Input: part model. Units: mm. Frame: model coordinates. A direction names the side the tool comes from. Coordinates: 2 decimals unless noted, no trailing zeros. Order: outer loops, then holes, each group sorted by start corner. A loop starts at its lowest first (then second) coordinate and runs counter-clockwise, first axis right, second up.
from build123d import *

# Parameters (mm, degrees)
BOSS_EXTRUDE1_DEPTH = 100
FILLET1_R           = 1
SKETCH2_R           = 2.5
CUT_EXTRUDE1_DEPTH  = 102.7840852
CUT_EXTRUDE2_DEPTH  = 102.7840852


with BuildPart() as part:
    # Sketch1 → Boss-Extrude1 (new body)
    with BuildSketch(Plane.XY):
        Polygon((0, 0), (18, 0), (18, 3), (3, 3), (3, 9), (0, 9), align=None)
    extrude(amount=BOSS_EXTRUDE1_DEPTH)

    # Fillet1
    fillet1_edges = [part.edges().sort_by_distance(p)[0] for p in [
        (3, 9, 50),
        (3, 3, 50),
        (18, 3, 50),
    ]]
    fillet(fillet1_edges, radius=FILLET1_R)

    # Sketch2 → Cut-Extrude1 (cut, through all)
    with BuildSketch(Plane(origin=(0, 3, 0), x_dir=(1, 0, 0), z_dir=(0, 1, 0))):
        with Locations(Location((10.5, -25, 0), (0, 0, 180))):
            Circle(SKETCH2_R)
        with Locations(Location((10.5, -75, 0), (0, 0, 180))):
            Circle(SKETCH2_R)
    extrude(amount=-CUT_EXTRUDE1_DEPTH, mode=Mode.SUBTRACT)

    # Sketch3 → Cut-Extrude2 (cut, through all)
    with BuildSketch(Plane(origin=(0, 3, 0), x_dir=(1, 0, 0), z_dir=(0, 1, 0))):
        with BuildLine():
            Line((8, -72.5), (13, -72.5))
            ThreePointArc((13, -72.5), (15.5, -75), (13, -77.5))
            Line((13, -77.5), (8, -77.5))
            ThreePointArc((8, -77.5), (5.5, -75), (8, -72.5))
        make_face()
        with BuildLine():
            Line((8, -27.5), (13, -27.5))
            ThreePointArc((13, -27.5), (15.5, -25), (13, -22.5))
            Line((13, -22.5), (8, -22.5))
            ThreePointArc((8, -22.5), (5.5, -25), (8, -27.5))
        make_face()
    extrude(amount=-CUT_EXTRUDE2_DEPTH, mode=Mode.SUBTRACT)


solid = part.part
Item 1: Ray query, probe 1 along Z at (x, y) = (11.5, 2.25); probe 2 along Y at (x, z) = (9.5, 87). Return the intervals inside material, ascending.
Response values:
probe 1: z = 0 to 22.5, 27.5 to 72.5, 77.5 to 100
probe 2: y = 0 to 3
Item 2: Pin query (flat end, axial travel): pin 1 Ø10.5 at (x, z) = (12, 40) entering from +Y; pin 2 Ø3 at (y, z) = (6.5, 55) entering from +X. Return the tip coordinate at first contact, or that it passes through.
Response values:
pin 1: stops at y = 3
pin 2: stops at x = 3
Item 3: Cut plane D-D on x = 6.5. Return loops of the section in (y, z).
Response values:
outline: (0, 0) - (3, 0) - (3, 23) - (0, 23) - close; (0, 27) - (3, 27) - (3, 73) - (0, 73) - close; (0, 77) - (3, 77) - (3, 100) - (0, 100) - close
Item 4: Access query for faces 5 (the face through (10, 2, 72.5)), 6 (the face through (11, 3, 49)), 7 (the face through (6.9, 2.6, 100)). Directions: +Z, -Z, +X, -X, +Y, -Y. A direction counts if a zero-diameter tool reaches every point of the face in a straight line with its end or side. Return the directions, or none.
Response values:
face 5: +Y, -Y
face 6: +Z, -Z, +X, +Y
face 7: +Z, +X, -X, +Y, -Y
Item 5: Cut plane A-A on z = 25. Return loops of the section in (x, y).
Response values:
outline: (0, 0) - (5.5, 0) - (5.5, 3) - (4, 3) arc R1 cw to (3, 4) - (3, 8) arc R1 ccw to (2, 9) - (0, 9) - close; (15.5, 0) - (18, 0) - (18, 2) arc R1 ccw to (17, 3) - (15.5, 3) - close
Item 6: Cut plane B-B on x = 11.5. Return loops of the section in (y, z), then the cut area to 3 significant figures.
Response values:
outline: (0, 0) - (3, 0) - (3, 22.5) - (0, 22.5) - close; (0, 27.5) - (3, 27.5) - (3, 72.5) - (0, 72.5) - close; (0, 77.5) - (3, 77.5) - (3, 100) - (0, 100) - close
area: 270 mm2
Item 7: Draft query along Z for faces 1 (the face through (15.5, 1.5, 74.9)), 2 (the face through (18, 1, 49)), 3 (the face through (10, 2, 27.5)), 4 (the face through (6.9, 2.6, 0)). Return one class per face: pulls with the +Z half, pulls with the -Z half, needs draft (parallel to the pull), parting line crosses it, or undercut.
Response values:
face 1: undercut
face 2: needs draft
face 3: undercut
face 4: pulls with the -Z half
Item 8: Cut plane C-C on z = 64.5. Return loops of the section in (x, y), then the cut area to 3 significant figures.
Response values:
outline: (0, 0) - (18, 0) - (18, 2) arc R1 ccw to (17, 3) - (4, 3) arc R1 cw to (3, 4) - (3, 8) arc R1 ccw to (2, 9) - (0, 9) - close
area: 71.8 mm2
